from build123d import *

# Parameters (mm, degrees)
SKETCH1_W           = 88
SKETCH1_H           = 160
BOSS_EXTRUDE1_DEPTH = 10
SKETCH2_W           = 88
SKETCH2_H           = 15
BOSS_EXTRUDE2_DEPTH = 15
SKETCH3_R           = 7.5
CUT_EXTRUDE1_DEPTH  = 88
FILLET1_R           = 10
SKETCH4_W           = 40
SKETCH4_H           = 65
CUT_EXTRUDE2_DEPTH  = 10
FILLET2_R           = 5
FILLET3_R           = 5
BOSS_EXTRUDE4_DEPTH = 30


with BuildPart() as part:
    # Sketch1 → Boss-Extrude1 (new body)
    with BuildSketch(Plane(origin=(0, 0, 0), x_dir=(1, 0, 0), z_dir=(0, 1, 0))):
        with Locations((44, 80)):
            Rectangle(SKETCH1_W, SKETCH1_H)
    extrude(amount=BOSS_EXTRUDE1_DEPTH)

    # Sketch2 → Boss-Extrude2 (add)
    with BuildSketch(Plane(origin=(0, 10, 0), x_dir=(1, 0, 0), z_dir=(0, 1, 0))):
        with Locations((44, 7.5)):
            Rectangle(SKETCH2_W, SKETCH2_H)
    extrude(amount=BOSS_EXTRUDE2_DEPTH)

    # Sketch3 → Cut-Extrude1 (cut)
    with BuildSketch(Plane(origin=(88, 0, 0), x_dir=(0, 0, -1), z_dir=(1, 0, 0))):
        with Locations((15, 17.5)):
            Circle(SKETCH3_R)
    extrude(amount=-CUT_EXTRUDE1_DEPTH, mode=Mode.SUBTRACT)

    # Fillet1
    # the kernel refuses this fillet: 10 mm, written as the material it takes off along each edge
    with BuildSketch(Plane(origin=(-25, 25, 0), x_dir=(0, -1, 0), z_dir=(1, 0, 0))) as fillet1_piece_1:
        with BuildLine():
            CenterArc((FILLET1_R, FILLET1_R), FILLET1_R, 180, 90)
            Line((0, FILLET1_R), (0, 0))
            Line((0, 0), (FILLET1_R, 0))
        make_face()
    extrude(amount=138, mode=Mode.SUBTRACT)
    with BuildSketch(Plane(origin=(-25, 0, 0), x_dir=(0, 1, 0), z_dir=(1, 0, 0))) as fillet1_piece_2:
        with BuildLine():
            CenterArc((FILLET1_R, -FILLET1_R), FILLET1_R, 90, 90)
            Line((0, -FILLET1_R), (0, 0))
            Line((0, 0), (FILLET1_R, 0))
        make_face()
    extrude(amount=138, mode=Mode.SUBTRACT)
    with BuildSketch(Plane(origin=(88, -25, 0), x_dir=(-1, 0, 0), z_dir=(0, 1, 0)), Plane(origin=(0, 50, 0), x_dir=(1, 0, 0), z_dir=(0, -1, 0))) as fillet1_piece_3:
        with BuildLine():
            CenterArc((FILLET1_R, -FILLET1_R), FILLET1_R, 90, 90)
            Line((0, -FILLET1_R), (0, 0))
            Line((0, 0), (FILLET1_R, 0))
        make_face()
    extrude(amount=75, mode=Mode.SUBTRACT)

    # Sketch4 → Cut-Extrude2 (cut)
    with BuildSketch(Plane(origin=(0, 10, 0), x_dir=(1, 0, 0), z_dir=(0, 1, 0))):
        with Locations((44, 127.5)):
            Rectangle(SKETCH4_W, SKETCH4_H)
    extrude(amount=-CUT_EXTRUDE2_DEPTH, mode=Mode.SUBTRACT)

    # Fillet2
    fillet2_edges = [part.edges().sort_by_distance(p)[0] for p in [
        (64, 5, -95),
        (24, 5, -95),
        (24, 5, -160),
        (64, 5, -160),
    ]]
    fillet(fillet2_edges, radius=FILLET2_R)

    # Fillet3
    fillet3_edges = [part.edges().sort_by_distance(p)[0] for p in [
        (0, 5, -160),
        (88, 5, -160),
    ]]
    fillet(fillet3_edges, radius=FILLET3_R)

    # Sketch5 → Boss-Extrude4 (add)
    with BuildSketch(Plane.ZY):
        Polygon((-70, 10), (-70, 0.2), (-49.5, 3.3), (-49.5, 6.9), align=None)
    boss_extrude4 = extrude(amount=BOSS_EXTRUDE4_DEPTH)

    # Mirror1: Boss-Extrude4 across plane
    add(boss_extrude4.mirror(Plane(origin=(44, 0, 0), x_dir=(0, 0, 1), z_dir=(1, 0, 0))))


solid = part.part
Geometry check sheet. Reference: the model listing, model coordinates, mm. A direction names the side the tool comes from. Give positions to 0.01 mm unless a question says otherwise; leave off trailing zeros. Loops run counter-clockwise (first coordinate to the right, second up) from the corner with the lowest first, then second, coordinate; pieces in that order, holes last.
(1) Section check C-C on z = -37.5. Record the cut outline in (x, y), then the cut area to 3 significant figures.
From the geometry:
outline: (0, 0) - (88, 0) - (88, 10) - (0, 10) - close
area: 880 mm2
(2) Depth check by flat-ended pin: pin 1 Ø4 at (x, z) = (59.5, -75.5) entering from -Y; pin 2 Ø1.5 at (x, y) = (6.5, 22.5) entering from -Z; pin 3 Ø8 at (y, z) = (3, -136.5) entering from +X; pin 4 Ø3 at (x, y) = (101, 5) entering from +Z. Enter the tip coordinate at first touch or a pass-through.
From the geometry:
pin 1: stops at y = 0
pin 2: stops at z = -10.18
pin 3: stops at x = 88
pin 4: stops at z = -49.5
(3) Thickness scan on L1, parallel to X at y = 1.5, z = -149; L2, parallel to Y at x = 81.5, z = -152.5; L3, parallel to X at y = 6, z = -37. Record the ranges inside material, lowest first.
From the geometry:
L1: x = 0 to 24, 64 to 88
L2: y = 0 to 10
L3: x = 0 to 88
(4) Section check A-A on z = -108. Record the cut outline in (x, y).
From the geometry:
outline: (0, 0) - (24, 0) - (24, 10) - (0, 10) - close; (64, 0) - (88, 0) - (88, 10) - (64, 10) - close
(5) Section check B-B on x = 37. Record the cut outline in (y, z), then the cut area to 3 significant figures.
From the geometry:
outline: (0, -95) - (10, -95) - (10, -15) arc R7.5 cw to (25, -15) - (25, -10) arc R10 ccw to (15, 0) - (10, 0) arc R10 ccw to (0, -10) - close
area: 1,040 mm2
(6) Release check for a two-part mould opening along Y. For faces 1 (the flat face through (-14.79, 8.43, -59.61)), 2 (the flat face through (-14.79, 1.73, -59.89)), 3 (the flat face through (12, 5, -160)), 4 (the cylindrical face through (44.62, 17.66, -7.5)) record: released by +Y, released by -Y, zero draft, split by the parting line, or undercut.
From the geometry:
face 1: released by +Y
face 2: released by -Y
face 3: zero draft
face 4: undercut
(7) Section check D-D on x = -6.5. Record the cut outline in (y, z).
From the geometry:
outline: (0.2, -70) - (10, -70) - (6.9, -49.5) - (3.3, -49.5) - close
(8) Set-up check for faces 5 (the cylindrical face through (25, 5, -97)), 6 (the flat face through (-15, 5, -49.5)), 7 (the flat face through (-15, 5, -70)): record each of +Z, -Z, +X, -X, +Y, -Y from which the full face is reachable in a straight line by a thin tool's end or side.
From the geometry:
face 5: -Z, +Y, -Y
face 6: +Z, -X, +Y, -Y
face 7: -Z, -X, +Y, -Y
